```python
from build123d import *

# Parameters (mm, degrees)
F0_R     = 3.1
F1_DEPTH = 3.175


with BuildPart() as f1:
    # F0 (on Front) → F1 (new body)
    with BuildSketch(Plane.XZ):
        with BuildLine():
            ThreePointArc((40, 2.5), (38.535534, 6.035534), (35, 7.5))
            Line((35, 7.5), (-35, 7.5))
            ThreePointArc((-35, 7.5), (-38.535534, 6.035534), (-40, 2.5))
            Line((-40, 2.5), (-40, -2.5))
            ThreePointArc((-40, -2.5), (-38.535534, -6.035534), (-35, -7.5))
            Line((-35, -7.5), (35, -7.5))
            ThreePointArc((35, -7.5), (38.535534, -6.035534), (40, -2.5))
            Line((40, -2.5), (40, 2.5))
        make_face()
        with Locations((-30, 0)):
            Circle(F0_R, mode=Mode.SUBTRACT)
        with BuildLine():
            ThreePointArc((28.289735, -2.674999), (27.215156, -1.524883), (26.825, 0))
            ThreePointArc((26.825, 0), (31.524883, 2.784844), (31.710265, -2.674999))
            Line((31.710265, -2.674999), (28.289735, -2.674999))
        make_face(mode=Mode.SUBTRACT)
    extrude(amount=F1_DEPTH)


solid = f1.part
```
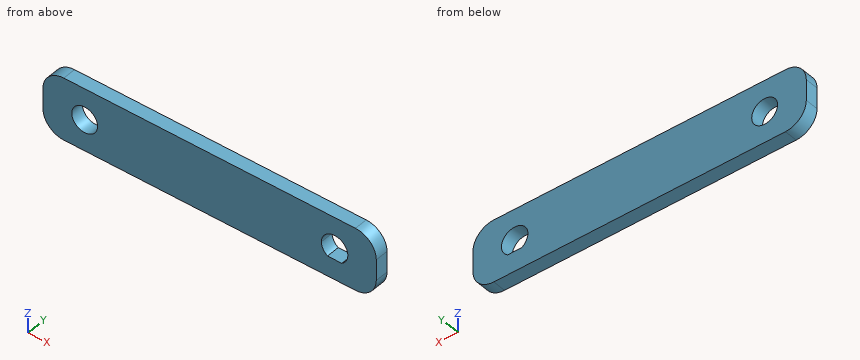
Can you work these out from the model? Positions are in its coordinate system, mm. Give positions to 0.01 mm unless a question says otherwise; leave off trailing zeros. Order: outer loops, then holes, each group sorted by start corner. A loop starts at its lowest first (then second) coordinate and runs counter-clockwise, first axis right, second up. Notation, with made-up numbers: (-1.5, 37) - (19.5, 37) arc R19 cw to (19.5, 43) - close; hole circle Ø3 at (83, 63). An arc over 180 degrees is marked (long way). Use a Markdown table: item, result. Add a question column.
Q1. If we section it at D-D on x = 30: Write out the boundary of the cut face in (y, z) (3 decimals), plus the area to 3 significant figures.
Q2. I'm going to push flat-ended pins straight in: pin 1 (5 mm diameter, centred on x = 30, z = 0, fed in from -Y); pin 2 (1.5 mm diameter, centred on y = -2, z = 4, fed in from +X). Where does each tip first touch, or does it pass through?
Q3. If we section it at C-C on z = -1: Write out the boundary of the cut face in (x, y) (3 decimals).
Q4. If we section it at A-A on y = -1.15: Write out the boundary of the cut face in (x, z) (3 decimals).
Q5. If we section it at B-B on x = -30: Write out the boundary of the cut face in (y, z) (3 decimals).
Q6. Please list where these lines run through material, in increasing order: line 1 along Z through (x, y) = (30, -1.15) (3 decimals); line 2 along Z through (x, y) = (-30, -0.65); line 3 along X through (y, z) = (-2.15, -2).
Answers follow:
| question | item | result |
|---|---|---|
| 1 | outline | (-3.175, -7.5) - (0, -7.5) - (0, -2.675) - (-3.175, -2.675) - close; (-3.175, 3.175) - (0, 3.175) - (0, 7.5) - (-3.175, 7.5) - close |
| 1 | area | 29.1 mm^2 |
| 2 | pin 1 | passes through |
| 2 | pin 2 | stops at x = 39.94 |
| 3 | outline | (-40, -3.175) - (-32.934, -3.175) - (-32.934, 0) - (-40, 0) - close; (-27.066, -3.175) - (26.987, -3.175) - (26.987, 0) - (-27.066, 0) - close; (33.013, -3.175) - (40, -3.175) - (40, 0) - (33.013, 0) - close |
| 4 | outline | (-40, -2.5) arc R5 ccw to (-35, -7.5) - (35, -7.5) arc R5 ccw to (40, -2.5) - (40, 2.5) arc R5 ccw to (35, 7.5) - (-35, 7.5) arc R5 ccw to (-40, 2.5) - close; hole circle Ø6.2 at (-30, 0); hole (26.825, 0) arc R3.175 ccw to (28.29, -2.675) - (31.71, -2.675) arc R3.175 ccw (long way) to start |
| 5 | outline | (-3.175, -7.5) - (0, -7.5) - (0, -3.1) - (-3.175, -3.1) - close; (-3.175, 3.1) - (0, 3.1) - (0, 7.5) - (-3.175, 7.5) - close |
| 6 | line 1 | z = -7.5 to -2.675, 3.175 to 7.5 |
| 6 | line 2 | z = -7.5 to -3.1, 3.1 to 7.5 |
| 6 | line 3 | x = -40 to -32.37, -27.63 to 27.53, 32.47 to 40 |
